Can you work these out from the model? Positions are in its coordinate system, mm. A direction names the side the tool comes from. Round coordinates to 2 decimals unless told otherwise and drop trailing zeros. Order: outer loops, then holes, each group sorted by start corner. A loop starts at its lowest first (then second) coordinate and runs counter-clockwise, first axis right, second up. Notation, with made-up numbers: M 39.5,-2.75 L 83.5,-2.75 A15 ccw 83.5,15.25 Z; hole C 40,42.25 d7. An arc over 180 degrees is marked long. Answer as a JSON object with one key per item and string values. Group by question number.
from build123d import *

# Parameters (mm, degrees)
F2_SIZE = 0.79375
F3_SIZE = 0.79375


with BuildPart() as f1:
    # F0 (on Front) → F1 (revolve)
    with BuildSketch(Plane.XZ):
        Polygon((0, 11.1125), (0, 0), (203.2, 0), (203.2, 6.35), (190.5, 6.35), (190.5, 7.9375), (109.599779, 11.1125), align=None)
    revolve(axis=Axis((101.6, 0, 0), (1, 0, 0)))

    # F2
    f2_edges = [f1.edges().sort_by_distance(p)[0] for p in [
        (190.5, 0, -7.9375),
    ]]
    chamfer(f2_edges, length=F2_SIZE)

    # F3
    f3_edges = [f1.edges().sort_by_distance(p)[0] for p in [
        (203.2, 0, -6.35),
    ]]
    chamfer(f3_edges, length=F3_SIZE)


solid = f1.part
Item 1: On a 3-axis mill with a long thin cutter (end or side, diameter ignored), from which of +Z, -Z, +X, -X, +Y, -Y can I reach the whole of each face in a straight line? I mean faces 1 (the face through (203.2, 0, 0)), 2 (the face through (196.37, 6.2, -1.38)). Say none if no direction works.
Item 2: I need wall thicknesses on line 1 (X direction, y = -2.25, z = 6.75); line 2 (Z direction, x = 97.5, y = -0.75); line 3 (X direction, y = 3.75, z = 5). Which ranges of each line are inside material? Lowest first, please.
Item 3: I'm going to push flat-ended pins straight in: pin 1 Ø4 at (x, z) = (147, 0.5) entering from -Y; pin 2 Ø6 at (x, z) = (136, -2) entering from -Y; pin 3 Ø6 at (x, z) = (24.5, -5.5) entering from -Y. Where does each tip first touch, or does it pass through?
Item 4: Suppose I cut it at C-C, the plane x = 84.5. Write out the boundary of the cut face in (y, z) (1 decimal).
Item 5: Suppose I cut it at A-A, the plane z = 0. Write out the boundary of the cut face in (x, y).
Computed:
{
 "1": {"face 1": "+Z, -Z, +X, +Y, -Y", "face 2": "+X"},
 "2": {"line 1": "x = 0 to 190.5", "line 2": "z = -11.09 to 11.09", "line 3": "x = 0 to 202.51"},
 "3": {"pin 1": "stops at y = -9.72", "pin 2": "stops at y = -10.17", "pin 3": "stops at y = -10.83"},
 "4": {"outline": "C 0,0 d22.2"},
 "5": {"outline": "M 0,-11.11 L 109.6,-11.11 L 189.71,-7.97 L 190.5,-7.14 L 190.5,-6.35 L 202.41,-6.35 L 203.2,-5.56 L 203.2,5.56 L 202.41,6.35 L 190.5,6.35 L 190.5,7.14 L 189.71,7.97 L 109.6,11.11 L 0,11.11 Z"}
}
